from build123d import *

# Parameters (mm, degrees)
ESQUISSE1_W             = 93
ESQUISSE1_H             = 93
BOSS_EXTRU_1_DEPTH      = 5
ESQUISSE2_W             = 53
ESQUISSE2_H             = 53
BOSS_EXTRU_2_DEPTH      = 48
ESQUISSE3_W             = 43
ESQUISSE3_H             = 43
ENL_V_MAT_EXTRU_1_DEPTH = 49
ENL_V_MAT_EXTRU_2_REACH = 55
ESQUISSE4_R             = 11.1
ENL_V_MAT_EXTRU_3_REACH = 7
ESQUISSE5_R             = 1.5
ESQUISSE7_W             = 10
ESQUISSE7_H             = 13
ENL_V_MAT_EXTRU_4_DEPTH = 10


with BuildPart() as part:
    # Esquisse1 → Boss.-Extru.1 (new body)
    with BuildSketch(Plane.XY):
        with Locations((25.019689463, -26.276315789)):
            Rectangle(ESQUISSE1_W, ESQUISSE1_H)
    extrude(amount=BOSS_EXTRU_1_DEPTH)

    # Esquisse2 → Boss.-Extru.2 (add)
    with BuildSketch(Plane.XY.offset(5)):
        with Locations((25.01969205, -26.276318376)):
            Rectangle(ESQUISSE2_W, ESQUISSE2_H)
    extrude(amount=BOSS_EXTRU_2_DEPTH)

    # Esquisse3 → Enlèv. mat.-Extru.1 (cut)
    with BuildSketch(Plane(origin=(0, 0, 0), x_dir=(-1, 0, 0), z_dir=(0, 0, -1))):
        with Locations((-25.019689463, -26.276315789)):
            Rectangle(ESQUISSE3_W, ESQUISSE3_H)
    extrude(amount=-ENL_V_MAT_EXTRU_1_DEPTH, mode=Mode.SUBTRACT)

    # Esquisse4 → Enlèv. mat.-Extru.2 (cut, up to next)
    with BuildSketch(Plane.XY.offset(53), mode=Mode.PRIVATE) as enl_v_mat_extru_2_sk1:
        with Locations((25.01969205, -26.276318376)):
            Circle(ESQUISSE4_R)
    enl_v_mat_extru_2_tool1 = extrude(enl_v_mat_extru_2_sk1.sketch, amount=-ENL_V_MAT_EXTRU_2_REACH, mode=Mode.PRIVATE) & part.part
    add(enl_v_mat_extru_2_tool1.solids().sort_by_distance((25.019692, -26.276318, 53))[0], mode=Mode.SUBTRACT)

    # Esquisse5 → Enlèv. mat.-Extru.3 (cut, up to next)
    with BuildSketch(Plane.XY.offset(5), mode=Mode.PRIVATE) as enl_v_mat_extru_3_sk1:
        with Locations((61.519689463, -62.776315789)):
            Circle(ESQUISSE5_R)
    enl_v_mat_extru_3_tool1 = extrude(enl_v_mat_extru_3_sk1.sketch, amount=-ENL_V_MAT_EXTRU_3_REACH, mode=Mode.PRIVATE) & part.part
    add(enl_v_mat_extru_3_tool1.solids().sort_by_distance((61.519689, -62.776316, 5))[0], mode=Mode.SUBTRACT)
    # Esquisse5 → Enlèv. mat.-Extru.3 (cut, up to next)
    with BuildSketch(Plane.XY.offset(5), mode=Mode.PRIVATE) as enl_v_mat_extru_3_sk2:
        with Locations((-11.480310537, -62.776315789)):
            Circle(ESQUISSE5_R)
    enl_v_mat_extru_3_tool2 = extrude(enl_v_mat_extru_3_sk2.sketch, amount=-ENL_V_MAT_EXTRU_3_REACH, mode=Mode.PRIVATE) & part.part
    add(enl_v_mat_extru_3_tool2.solids().sort_by_distance((-11.480311, -62.776316, 5))[0], mode=Mode.SUBTRACT)
    # Esquisse5 → Enlèv. mat.-Extru.3 (cut, up to next)
    with BuildSketch(Plane.XY.offset(5), mode=Mode.PRIVATE) as enl_v_mat_extru_3_sk3:
        with Locations((-11.480310537, 10.223684211)):
            Circle(ESQUISSE5_R)
    enl_v_mat_extru_3_tool3 = extrude(enl_v_mat_extru_3_sk3.sketch, amount=-ENL_V_MAT_EXTRU_3_REACH, mode=Mode.PRIVATE) & part.part
    add(enl_v_mat_extru_3_tool3.solids().sort_by_distance((-11.480311, 10.223684, 5))[0], mode=Mode.SUBTRACT)
    # Esquisse5 → Enlèv. mat.-Extru.3 (cut, up to next)
    with BuildSketch(Plane.XY.offset(5), mode=Mode.PRIVATE) as enl_v_mat_extru_3_sk4:
        with Locations((61.519689463, 10.223684211)):
            Circle(ESQUISSE5_R)
    enl_v_mat_extru_3_tool4 = extrude(enl_v_mat_extru_3_sk4.sketch, amount=-ENL_V_MAT_EXTRU_3_REACH, mode=Mode.PRIVATE) & part.part
    add(enl_v_mat_extru_3_tool4.solids().sort_by_distance((61.519689, 10.223684, 5))[0], mode=Mode.SUBTRACT)

    # Esquisse7 → Enlèv. mat.-Extru.4 (cut)
    with BuildSketch(Plane.XZ.offset(4.776315789)):
        with Locations((24.207318305, 6.5)):
            Rectangle(ESQUISSE7_W, ESQUISSE7_H)
    extrude(amount=-ENL_V_MAT_EXTRU_4_DEPTH, mode=Mode.SUBTRACT)


solid = part.part
Input: part model. Units: mm. Frame: model coordinates. A direction names the side the tool comes from. Give positions to 0.01 mm unless a question says otherwise; leave off trailing zeros. Write each loop counter-clockwise with the first axis right and the second up, starting at its lowest first coordinate (ties: lowest second). Pieces come first, ordered by that corner, then holes.
Q1. Set-up query: faces 4 (the face through (19.207, -1, 5)), 5 (the face through (24, 5.224, 3)), 6 (the face through (25, -52.776, 29)), 7 (the face through (25, 0.224, 29)). Return all of +Z, -Z, +X, -X, +Y, -Y with unobstructed straight access to the full face (end or side cutting, diameter ignored); none if empty.
Q2. Section B-B, the plane y = -1. Output: boundary loops of the cut face in (x, z).
Q3. First-contact query: P1, Ø5, axis at x = -11.48, y = 10.22, coming from the +Z side; P2, Ø1.5, axis at x = 25, y = -3.5, coming from the -Z side; P3, Ø5, axis at y = 0.5, z = 9, coming from the +X side. Flat tips, straight axial feed; report the tip coordinate or a pass-through.
Q4. Material intervals for probe 1 along X at (y, z) = (10, 2.5); probe 2 along X at (y, z) = (-46.5, 12); probe 3 along Y at (x, z) = (28.5, 46.5), sorted ascending.
Q5. Section C-C, the plane z = 11.5. Output: boundary loops of the cut face in (x, y), plus the area to 3 significant figures.
Q6. Section D-D, the plane y = -23.5. Output: boundary loops of the cut face in (x, z), plus the area to 3 significant figures.
Q7. Section A-A, the plane z = 29. Output: boundary loops of the cut face in (x, y), plus the area to 3 significant figures.
Q8. Pull-direction query (X, two-part tool) for faces 1 (the face through (61.32, -61.29, 2.54)), 2 (the face through (24.4, 5.4, 5)), 3 (the face through (-1.48, -27, 29)); classes: pulls with the +X half, pulls with the -X half, needs draft (parallel to the pull), parting line crosses it, or undercut.
Filled in:
1. face 4: -Z
1. face 5: +Z, -Z
1. face 6: +Z, +X, -X, -Y
1. face 7: +Z, +X, -X, +Y
2. outline: (-21.48, 0) - (19.21, 0) - (19.21, 13) - (29.21, 13) - (29.21, 0) - (71.52, 0) - (71.52, 5) - (51.52, 5) - (51.52, 53) - (-1.48, 53) - (-1.48, 5) - (-21.48, 5) - close
3. P1: stops at z = 5
3. P2: stops at z = 13
3. P3: stops at x = 51.52
4. probe 1: x = -21.48 to -12.96, -10 to 60.04, 63 to 71.52
4. probe 2: x = -1.48 to 3.52, 46.52 to 51.52
4. probe 3: y = -52.78 to -47.78, -4.78 to 0.22
5. outline: (-1.48, -52.78) - (51.52, -52.78) - (51.52, 0.22) - (29.21, 0.22) - (29.21, -4.78) - (46.52, -4.78) - (46.52, -47.78) - (3.52, -47.78) - (3.52, -4.78) - (19.21, -4.78) - (19.21, 0.22) - (-1.48, 0.22) - close
5. area: 910 mm2
6. outline: (-21.48, 0) - (3.52, 0) - (3.52, 49) - (14.27, 49) - (14.27, 53) - (-1.48, 53) - (-1.48, 5) - (-21.48, 5) - close; (35.77, 49) - (46.52, 49) - (46.52, 0) - (71.52, 0) - (71.52, 5) - (51.52, 5) - (51.52, 53) - (35.77, 53) - close
6. area: 816 mm2
7. outline: (-1.48, -52.78) - (51.52, -52.78) - (51.52, 0.22) - (-1.48, 0.22) - close; hole (3.52, -47.78) - (46.52, -47.78) - (46.52, -4.78) - (3.52, -4.78) - close
7. area: 960 mm2
8. face 1: undercut
8. face 2: needs draft
8. face 3: pulls with the -X half
